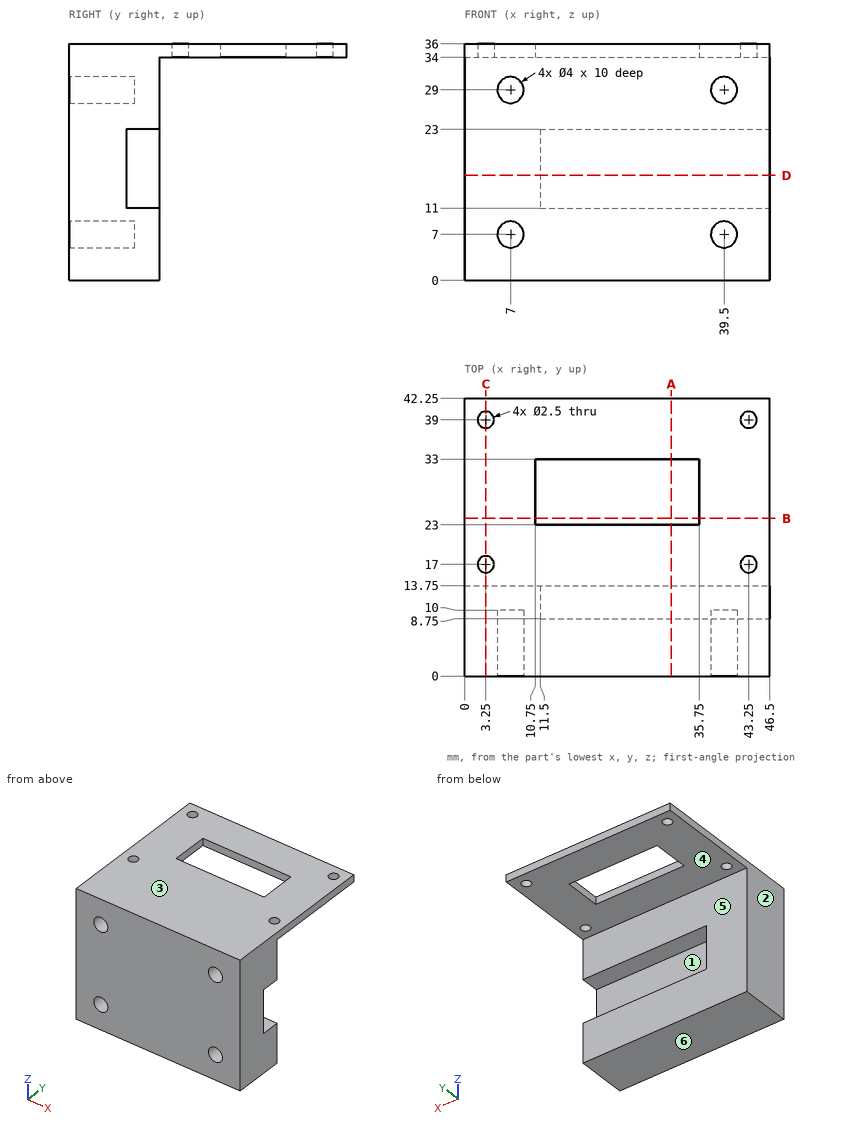
Answer from the drawing. Dimensions are ordinates in mm from the lowest x, y and z of the part. A direction names the side the tool comes from. Round coordinates to 2 decimals unless told otherwise and drop trailing zeros. Write each loop counter-clockwise with the first axis right and the second up, starting at its lowest first coordinate (ties: lowest second). Pieces come first, ordered by that corner, then holes. Notation, with made-up numbers: (34, 1.25) - (73, 1.25) arc R8 cw to (73, 5.25) - close; hole circle Ø1 at (82.25, 25). An arc over 180 degrees is marked (long way). Use a Markdown table: item, result.
(1) The part is cut by section D-D (z = 16). Write down the section's boundary in (x, y), then the cut area to 3 significant figures.
Reported:
| item | result |
|---|---|
| outline | (0, 0) - (46.5, 0) - (46.5, 8.75) - (11.5, 8.75) - (11.5, 13.75) - (0, 13.75) - close |
| area | 464 mm2 |
(2) Straight lines are drawn through the part: line 1 along X through (y, z) = (3, 7); line 2 along Z through (x, y) = (39, 5); line 3 along Z through (x, y) = (41, 2.5). For each, find the intervals that lie inside material, in ascending order. Write a range as [from, to].
Reported:
| item | result |
|---|---|
| line 1 | [0, 5], [9, 37.5], [41.5, 46.5] |
| line 2 | [0, 5.06], [8.94, 27.06], [30.94, 36] |
| line 3 | [0, 5.68], [8.32, 27.68], [30.32, 36] |
(3) The part is cut by section C-C (x = 3.25). Write down the section's boundary in (y, z), then the cut area to 3 significant figures.
Reported:
| item | result |
|---|---|
| outline | (0, 0) - (13.75, 0) - (13.75, 34) - (15.75, 34) - (15.75, 36) - (0, 36) - close; (18.25, 34) - (37.75, 34) - (37.75, 36) - (18.25, 36) - close; (40.25, 34) - (42.25, 34) - (42.25, 36) - (40.25, 36) - close |
| area | 542 mm2 |
(4) The part is cut by section B-B (y = 24). Write down the section's boundary in (x, z).
Reported:
| item | result |
|---|---|
| outline | (0, 34) - (10.75, 34) - (10.75, 36) - (0, 36) - close; (35.75, 34) - (46.5, 34) - (46.5, 36) - (35.75, 36) - close |
(5) The mould has two halves that part along Z. Classify the marked faces 1, 2, 3 and 4: released by +Z, released by -Z, zero draft, split by the parting line, or undercut.
Reported:
| item | result |
|---|---|
| face 1 | undercut |
| face 2 | zero draft |
| face 3 | released by +Z |
| face 4 | released by -Z |
(6) The part is cut by section A-A (x = 31.5). Write down the section's boundary in (y, z), then the cut area to 3 significant figures.
Reported:
| item | result |
|---|---|
| outline | (0, 0) - (13.75, 0) - (13.75, 11) - (8.75, 11) - (8.75, 23) - (13.75, 23) - (13.75, 34) - (23, 34) - (23, 36) - (0, 36) - close; (33, 34) - (42.25, 34) - (42.25, 36) - (33, 36) - close |
| area | 472 mm2 |
(7) Which of the six approach directions +Z, -Z, +X, -X, +Y, -Y give full straight-line access (tool end or side, diameter ignored) to the marked faces 5 and 6?
Reported:
| item | result |
|---|---|
| face 5 | -Z, +X, -X, +Y |
| face 6 | -Z, +X, -X, +Y, -Y |
(8) Each of these flat-tipped pins is pushed along its axis until it touches: pin 1 Ø4 at (y, z) = (12, 18.5) entering from +X; pin 2 Ø14 at (x, y) = (35, 28) entering from -Z; pin 3 Ø6.5 at (x, z) = (39.5, 7) entering from +Y; pin 4 Ø2 at (x, y) = (43.25, 39) entering from +Z (3 decimals). Where does it stop, or does it pass through?
Reported:
| item | result |
|---|---|
| pin 1 | x = 11.5 |
| pin 2 | z = 34 |
| pin 3 | y = 13.75 |
| pin 4 | through |
